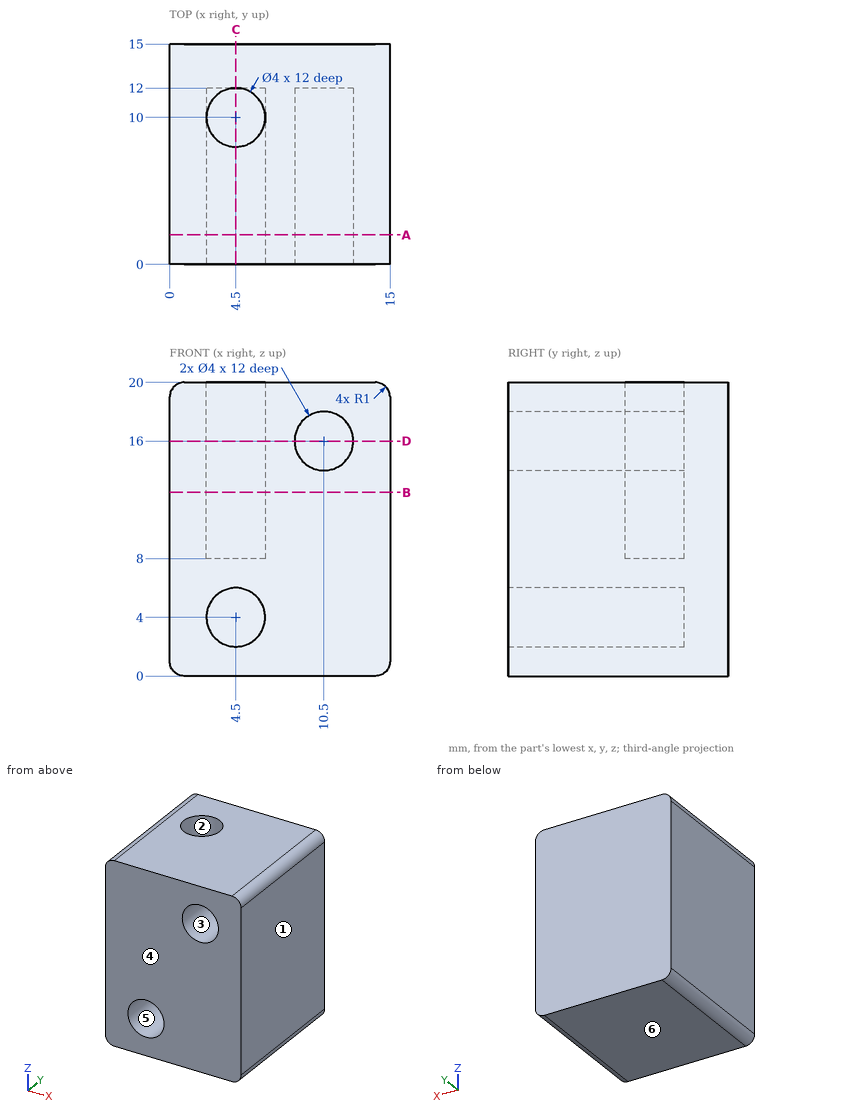
Could you check a few things on this drawing? It's one solid part, dimensions in mm from its lowest x, y, z. A direction names the side the tool comes from. Round coordinates to 2 decimals unless told otherwise and drop trailing zeros. Loops run counter-clockwise (first coordinate to the right, second up) from the corner with the lowest first, then second, coordinate; pieces in that order, holes last. Notation, with made-up numbers: M 22,31.5 L 56,31.5 A12 cw 56,38.5 Z; hole C -34,79.25 d3. An arc over 180 degrees is marked long. Write item = value, one per line. Start each with the question number.
(1) I'm going to push a flat-ended pin straight in: P1, Ø3, axis at x = 10.5, z = 16, coming from the -Y side. Where does the tip first touch, or does it pass through?
(2) If we mould it in two halves opening along X, with no side actions, what happens to the marked faces 1, 2, 3 and 4? For each: released by +X, released by -X, zero draft, split by the parting line, or undercut.
(3) Which directions (+Z, -Z, +X, -X, +Y, -Y) give clear straight access to the entire face, cutting with the end or side of a thin tool? Please do the marked faces 5 and 6.
(4) Suppose I cut it at B-B on z = 12.5. Write out the boundary of the cut face in (x, y), plus the area to 3 significant figures.
(5) Suppose I cut it at C-C on x = 4.5. Write out the boundary of the cut face in (y, z).
(6) Suppose I cut it at D-D on z = 16. Write out the boundary of the cut face in (x, y), plus the area to 3 significant figures.
(7) Suppose I cut it at A-A on y = 2. Write out the boundary of the cut face in (x, z).
(8) I need wall thicknesses on line 1 along Y through (x, z) = (4.5, 12.25); line 2 along X through (y, z) = (3.5, 16); line 3 along Y through (x, z) = (10.5, 16.25). Which ranges of each line are inside material? Lowest first, please.
Answer block:
q1.P1 = 12
q2.face_1 = released by +X
q2.face_2 = undercut
q2.face_3 = undercut
q2.face_4 = zero draft
q3.face_5 = -Y
q3.face_6 = -Z, +X, -X, +Y, -Y
q4.outline = M 0,0 L 15,0 L 15,15 L 0,15 Z; hole C 4.5,10 d4
q4.area = 212 mm²
q5.outline = M 0,0 L 15,0 L 15,20 L 12,20 L 12,8 L 8,8 L 8,20 L 0,20 L 0,6 L 12,6 L 12,2 L 0,2 Z
q6.outline = M 0,0 L 8.5,0 L 8.5,12 L 12.5,12 L 12.5,0 L 15,0 L 15,15 L 0,15 Z; hole C 4.5,10 d4
q6.area = 164 mm²
q7.outline = M 0,1 A1 ccw 1,0 L 14,0 A1 ccw 15,1 L 15,19 A1 ccw 14,20 L 1,20 A1 ccw 0,19 Z; hole C 4.5,4 d4; hole C 10.5,16 d4
q8.line_1 = 0 to 8, 12 to 15
q8.line_2 = 0 to 8.5, 12.5 to 15
q8.line_3 = 12 to 15
